Geometry: final body of the model. Coordinates: model frame, mm. A direction names the side the tool comes from. Give positions to 0.01 mm unless a question says otherwise; leave off trailing zeros. Loops run counter-clockwise (first coordinate to the right, second up) from the corner with the lowest first, then second, coordinate; pieces in that order, holes last.
```python
from build123d import *

# Parameters (mm, degrees)
SKETCH_24_R         = 7.643312102
BOSS_EXTRUDE1_DEPTH = 4
SKETCH3_W           = 5
SKETCH3_H           = 1.5
SKETCH3_W_2         = 3
SKETCH5_R           = 4.458598726
BOSS_EXTRUDE2_DEPTH = 4
SKETCH6_W           = 4
SKETCH6_H           = 1.5
SKETCH6_W_2         = 3
CUT_EXTRUDE2_DEPTH  = 2
CUT_EXTRUDE3_DEPTH  = 2
BOSS_EXTRUDE4_START = 3
SKETCH10_R          = 0.5
BOSS_EXTRUDE4_DEPTH = 3
CHAMFER1_START      = -4
CHAMFER1_2_DEPTH    = 4


with BuildPart() as part:
    # Sketch 24 → Boss-Extrude1 (new body)
    with BuildSketch(Plane(origin=(0, 0, 0), x_dir=(1, 0, 0), z_dir=(0, 1, 0))):
        with Locations(Location((0, 0, 0), (0, 0, 270))):
            Circle(SKETCH_24_R)
    extrude(amount=BOSS_EXTRUDE1_DEPTH)

    # Sketch3 → Revolve1 (revolve)
    with BuildSketch(Plane.XY, mode=Mode.PRIVATE) as revolve1_sk:
        with Locations((-10.143312102, 0.75)):
            Rectangle(SKETCH3_W, SKETCH3_H)
        with Locations((-9.143312102, 3.25)):
            Rectangle(SKETCH3_W_2, SKETCH3_H)
    revolve(revolve1_sk.sketch.rotate(Axis((0, 4, 0), (0, -1, 0)), 270), axis=Axis((0, 4, 0), (0, -1, 0)))

    # Sketch5 → Boss-Extrude2 (add)
    with BuildSketch(Plane(origin=(0, 4, 0), x_dir=(1, 0, 0), z_dir=(0, 1, 0))):
        with Locations(Location((0, 0, 0), (0, 0, 270))):
            Circle(SKETCH5_R)
    extrude(amount=BOSS_EXTRUDE2_DEPTH)

    # Sketch6 → Revolve2 (revolve)
    with BuildSketch(Plane.XY, mode=Mode.PRIVATE) as revolve2_sk:
        with Locations((-6.458598726, 7.25)):
            Rectangle(SKETCH6_W, SKETCH6_H)
        with Locations((-5.958598726, 4.75)):
            Rectangle(SKETCH6_W_2, SKETCH6_H)
    revolve(revolve2_sk.sketch.rotate(Axis((0, 4, 0), (0, -1, 0)), 270), axis=Axis((0, 4, 0), (0, -1, 0)))

    # Sketch8 → Cut-Extrude2 (cut)
    with BuildSketch(Plane.XZ):
        with BuildLine():
            Line((-0.7, 10), (-1.5, 10))
            ThreePointArc((-1.5, 10), (-2.5, 9), (-1.5, 8))
            Line((-1.5, 8), (-0.7, 8))
            Line((-0.7, 8), (-0.7, 10))
        make_face()
        with BuildLine():
            Line((1.5, 10), (0.7, 10))
            Line((0.7, 10), (0.7, 8))
            Line((0.7, 8), (1.5, 8))
            ThreePointArc((1.5, 8), (2.5, 9), (1.5, 10))
        make_face()
    extrude(amount=-CUT_EXTRUDE2_DEPTH, mode=Mode.SUBTRACT)

    # Sketch9 → Cut-Extrude3 (cut)
    with BuildSketch(Plane(origin=(0, 8, -8), x_dir=(-1, 0, 0), z_dir=(0, -1, 0))):
        with BuildLine():
            Line((-0.7, -1.2), (-1.5, -1.2))
            ThreePointArc((-1.5, -1.2), (-2.5, -2.2), (-1.5, -3.2))
            Line((-1.5, -3.2), (-0.7, -3.2))
            Line((-0.7, -3.2), (-0.7, -1.2))
        make_face()
        with BuildLine():
            Line((1.5, -1.2), (0.7, -1.2))
            Line((0.7, -1.2), (0.7, -3.2))
            Line((0.7, -3.2), (1.5, -3.2))
            ThreePointArc((1.5, -3.2), (2.5, -2.2), (1.5, -1.2))
        make_face()
    extrude(amount=CUT_EXTRUDE3_DEPTH, mode=Mode.SUBTRACT)

    # Sketch10 → Boss-Extrude4 (add)
    with BuildSketch(Plane.XZ.offset(BOSS_EXTRUDE4_START)):
        with BuildLine():
            Line((11.12894159, 6), (-11.12894159, 6))
            ThreePointArc((-11.12894159, 6), (-6.572693348, -10.800603829), (10.442822057, -7.127468582))
            ThreePointArc((10.442822057, -7.127468582), (12.080670499, -3.729710606), (12.643312102, 0))
            ThreePointArc((12.643312102, 0), (12.258874801, 3.094079752), (11.12894159, 6))
        make_face()
        with Locations(Location((-7.25, 0, 0), (0, 0, 270))):
            Circle(SKETCH10_R, mode=Mode.SUBTRACT)
        with Locations(Location((7.25, 0, 0), (0, 0, 270))):
            Circle(SKETCH10_R, mode=Mode.SUBTRACT)
    extrude(amount=-BOSS_EXTRUDE4_DEPTH)

    # Chamfer1: read off the stored shape, not the designer's step
    # Chamfer1 outline → Chamfer1 (revolve, cut)
    with BuildSketch(Plane.XY):
        Polygon((10.643312102, 3.5), (9.643312102, 2.5), (10.643312102, 2.5), align=None)
        Polygon((6.458598726, 5.5), (7.458598726, 4.5), (7.458598726, 5.5), align=None)
        Polygon((7.458598726, 6.5), (8.458598726, 6.5), (8.458598726, 7.5), align=None)
    revolve(axis=Axis((0, 0, 0), (0, 1, 0)), mode=Mode.SUBTRACT)

    # Chamfer1 2 outline → Chamfer1 2 (cut)
    with BuildSketch(Plane(origin=(0, 0, 0), x_dir=(1, 0, 0), z_dir=(0, 1, 0)).offset(CHAMFER1_START)):
        with BuildLine():
            ThreePointArc((11.12894159, -6), (11.349578809, -5.571391366), (11.553716625, -5.134683345))
            Line((11.553716625, -5.134683345), (8.663849742, -6))
            Line((8.663849742, -6), (11.12894159, -6))
        make_face()
        with BuildLine():
            Line((-11.12894159, -6), (-10.12894159, -6))
            Line((-10.12894159, -6), (-11.923354215, -4.205587374))
            ThreePointArc((-11.923354215, -4.205587374), (-11.561014862, -5.118229798), (-11.12894159, -6))
        make_face()
    extrude(amount=CHAMFER1_2_DEPTH, mode=Mode.SUBTRACT)


solid = part.part
```
Q1. Section query B-B, the plane y = 2. Return loops of the section in (x, z), and give its area (3 significant figures).
Q2. Section query A-A, the plane z = -5.8. State how many separate pieces and enclosed holes the cut face has, and give its area (3 significant figures).
Q3. Material intervals for probe 1 along Y at (x, z) = (-7.5, 2.25); probe 2 along Y at (x, z) = (-2.75, 8.75); probe 3 along Y at (x, z) = (-10.75, -0.5), sorted ascending.
Q4. Reachability of faces 5 (the face through (0, 6.5, 5)), 6 (the face through (6.762, -1.521, 0.108)), 7 (the face through (-1, -2, 6)), 8 (the face through (0, -3, -3)), 9 (the face through (-8.974, 3.754, 5.722)) from +Z, -Z, +X, -X, +Y, -Y: full face, straight path, thin tool, end or side. Return the list, or none.
Q5. Pin query (flat end, axial travel): pin 1 Ø0.9 at (x, y) = (-1.5, 7) entering from +Z; pin 2 Ø0.8 at (y, z) = (7, -5.5) entering from +X; pin 3 Ø6 at (x, y) = (-10, -2) entering from -Z. Return the tip coordinate at first contact, or that it passes through.
Q6. Mould query, pull axis Z, two halves, no side actions, for faces 1 (the face through (-11.01, -1.52, 5.12)), 2 (the face through (0.7, 7, -6)), 3 (the face through (-4.4, 5.5, -1.5)), 4 (the face through (-0.7, 1, 9)). Classes: +Z half, -Z half, draft (parallel to the pull), parting line (faces both ways), or undercut.
Resolved:
1. outline: circle Ø15.29 at (0, 0)
1. area: 184 mm2
2. separate pieces: 4
2. enclosed holes: 0
2. area: 161 mm2
3. probe 1: y = -3 to 1.5, 2.5 to 4, 6.87 to 8
3. probe 2: y = 0 to 1.5, 2.5 to 4
3. probe 3: y = -3 to 1.5
4. face 5: none
4. face 6: -Y
4. face 7: +Z, +X, -X, -Y
4. face 8: +Z, -Z, +X, -X, -Y
4. face 9: +Y
5. pin 1: stops at z = 8.28
5. pin 2: stops at x = 6.39
5. pin 3: stops at z = -10.53
6. face 1: +Z half
6. face 2: undercut
6. face 3: draft
6. face 4: undercut
